Check sheet for the modelled part. Datum: model origin and axes. Units: mm. A direction names the side the tool comes from. Round coordinates to 2 decimals unless told otherwise and drop trailing zeros. Write each loop counter-clockwise with the first axis right and the second up, starting at its lowest first coordinate (ties: lowest second). Pieces come first, ordered by that corner, then holes. Notation, with made-up numbers: (41.25, -32) -> (52.25, -32) arc R22 ccw to (52.25, -10) -> close; hole circle Ø11 at (6, 87.5). An arc over 180 degrees is marked (long way). Put each result on its own line as item: value. Start each with the question number.
from build123d import *
from build123d.topology import SkipClean

# Parameters (mm, degrees)
BOSS_EXTRU_1_DEPTH      = 5
ESQUISSE2_R             = 8
ENL_V_MAT_EXTRU_1_DEPTH = 4
ENL_V_MAT_EXTRU_2_DEPTH = 91.691785736
CHANFREIN1_SIZE         = 1


with BuildPart() as part:
    # Esquisse1 → Boss.-Extru.1 (new body)
    with BuildSketch(Plane.XY):
        with BuildLine():
            Line((-10, 0), (-10, 80))
            ThreePointArc((-10, 80), (0, 90), (10, 80))
            Line((10, 80), (10, 0))
            ThreePointArc((10, 0), (0, -10), (-10, 0))
        make_face()
    extrude(amount=BOSS_EXTRU_1_DEPTH)

    # Esquisse2 → Enlèv. mat.-Extru.1 (cut)
    with BuildSketch(Plane.XY.offset(5)):
        Circle(ESQUISSE2_R)
        with Locations((0, 80)):
            Circle(ESQUISSE2_R)
    extrude(amount=-ENL_V_MAT_EXTRU_1_DEPTH, mode=Mode.SUBTRACT)

    # Esquisse3 → Enlèv. mat.-Extru.2 (cut, through all)
    with SkipClean():  # the faces are left unmerged after this step: merging them gives an invalid solid
        with BuildSketch(Plane.XY.offset(5)):
            with BuildLine():
                Line((-4, 55), (-4, 25))
                ThreePointArc((-4, 25), (-5.244872469, 14.478769393), (-8.910741301, 4.538577912))
                ThreePointArc((-8.910741301, 4.538577912), (-9.72387302, 2.333729525), (-10, 0))
                Line((-10, 0), (-10, 80))
                ThreePointArc((-10, 80), (-9.72387302, 77.666270475), (-8.910741301, 75.461422088))
                ThreePointArc((-8.910741301, 75.461422088), (-5.244872469, 65.521230607), (-4, 55))
            make_face()
            with BuildLine():
                Line((4, 55), (4, 25))
                ThreePointArc((4, 25), (5.244872469, 14.478769393), (8.910741301, 4.538577912))
                ThreePointArc((8.910741301, 4.538577912), (9.72387302, 2.333729525), (10, 0))
                Line((10, 0), (10, 80))
                ThreePointArc((10, 80), (9.72387302, 77.666270475), (8.910741301, 75.461422088))
                ThreePointArc((8.910741301, 75.461422088), (5.244872469, 65.521230607), (4, 55))
            make_face()
        extrude(amount=-ENL_V_MAT_EXTRU_2_DEPTH, mode=Mode.SUBTRACT)

    # Chanfrein1
    chanfrein1_edges = [part.edges().sort_by_distance(p)[0] for p in [
        (-8, 0, 5),
        (-8, 80, 5),
    ]]
    chamfer(chanfrein1_edges, length=CHANFREIN1_SIZE)


solid = part.part
1. Section check C-C, the plane y = 70. Enter the section's corners in (x, z).
2. Access from +Z, -Z, +X, -X, +Y, -Y to the whole of each face (thin tool, end or side, straight path). Record for faces 4 (the flat face through (2, 40, 5)), 5 (the cylindrical face through (-1.73, -7.81, 2.52)), 6 (the flat face through (4, 40, 3)), 7 (the cylindrical face through (-5.21, 14.62, 2.54)).
3. Section check D-D, the plane y = 56.5. Enter the section's corners in (x, z), then the cut area to 3 significant figures.
4. Material ranges on L1, parallel to Y at x = 0, z = 2.2; L2, parallel to Y at x = -3, z = 3.3; L3, parallel to Z at x = -3.5, y = 77.5, recorded low to high. Write a range as [from, to].
5. Draft check along X on faces 1 (the cylindrical face through (-1.041, 87.932, 2.521)), 2 (the flat face through (-4, 40, 3)), 3 (the cylindrical face through (5.28, 65.67, 2.54)). Enter one of: released by +X, released by -X, zero draft, split by the parting line, or undercut.
6. Section check A-A, the plane x = 0. Enter the section's corners in (y, z).
7. Gauge pin test, flat ends, axial feed: P1, Ø2.5, axis at y = 33.5, z = 2, coming from the -X side; P2, Ø3, axis at x = 2, z = 4, coming from the -Y side. Record the tip position at first contact, or that the pin passes through.
8. Section check B-B, the plane z = 1.8. Enter the section's corners in (x, y).
Reply:
1. outline: (-6.57, 0) -> (6.57, 0) -> (6.57, 5) -> (-6.57, 5) -> close
2. face 4: +Z, +X, -X, +Y, -Y
2. face 5: +Z
2. face 6: +Z, -Z, +X
2. face 7: +Z, -Z, -X
3. outline: (-4.02, 0) -> (4.02, 0) -> (4.02, 5) -> (-4.02, 5) -> close
3. area: 40.2 mm2
4. L1: y = [-10, -8], [8, 72], [88, 90]
4. L2: y = [-9.54, -7.42], [7.42, 72.58], [87.42, 89.54]
4. L3: z = [0, 1]
5. face 1: undercut
5. face 2: released by -X
5. face 3: released by +X
6. outline: (-10, 0) -> (90, 0) -> (90, 5) -> (89, 5) -> (88, 4) -> (88, 1) -> (72, 1) -> (72, 4) -> (71, 5) -> (9, 5) -> (8, 4) -> (8, 1) -> (-8, 1) -> (-8, 4) -> (-9, 5) -> (-10, 5) -> close
7. P1: stops at x = -4
7. P2: stops at y = -9.99
8. outline: (-8.91, 4.54) arc R10 ccw (long way) to (8.91, 4.54) arc R45.08 cw to (4, 25) -> (4, 55) arc R45.08 cw to (8.91, 75.46) arc R10 ccw (long way) to (-8.91, 75.46) arc R45.08 cw to (-4, 55) -> (-4, 25) arc R45.08 cw to start; hole circle Ø16 at (0, 0); hole circle Ø16 at (0, 80)
